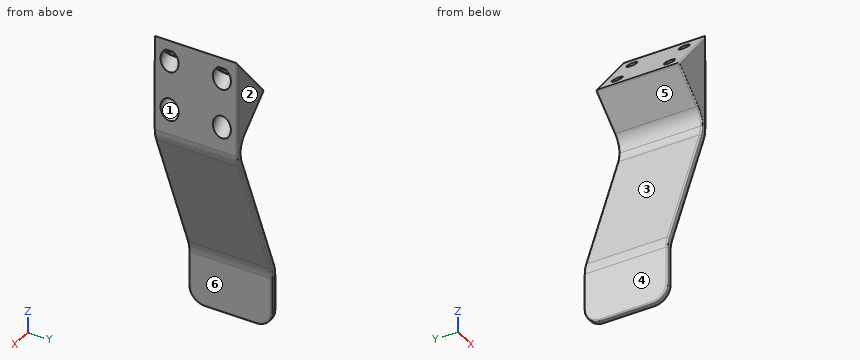
from build123d import *

# Parameters (mm, degrees)
SKETCH1_W           = 2
SKETCH1_H           = 25.4
SKETCH4_W           = 5
SKETCH4_H           = 25.4
CUT_EXTRUDE2_DEPTH  = 21
BOSS_EXTRUDE2_DEPTH = 25.4
BOSS_EXTRUDE4_DEPTH = 25.4
FILLET1_R           = 5
CUT_EXTRUDE3_DEPTH  = 26.4
SKETCH9_R           = 1.6
CUT_EXTRUDE4_DEPTH  = 2
SKETCH10_R          = 2.75
CUT_EXTRUDE5_DEPTH  = 59.842249491
FILLET2_R           = 10
FILLET5_R           = 6
FILLET3_R           = 0.4


with BuildPart() as part:
    # Sweep1: sweep along a path in Sketch2
    with BuildLine(Plane(origin=(0, 0, 0), x_dir=(1, 0, 0), z_dir=(0, 1, 0))) as sweep1_path:
        Line((22, 0), (22, 57.2))
        Line((22, 57.2), (4, 103.2))
        Line((4, 103.2), (4, 121.2))
    # Sketch1 → Sweep1 (sweep)
    with BuildSketch(Plane.XY):
        with Locations((22, 0)):
            Rectangle(SKETCH1_W, SKETCH1_H)
    sweep(path=sweep1_path.line, transition=Transition.RIGHT)

    # Sketch4 → Cut-Extrude2 (cut, through all)
    with BuildSketch(Plane(origin=(23, 0, 0), x_dir=(0, 0, -1), z_dir=(1, 0, 0))):
        with Locations((2.5, 0)):
            Rectangle(SKETCH4_W, SKETCH4_H)
    extrude(amount=-CUT_EXTRUDE2_DEPTH, mode=Mode.SUBTRACT)

    # Sketch5 → Boss-Extrude2 (add, through all)
    with BuildSketch(Plane.XZ.offset(12.7)):
        Polygon((21, -42.561313548), (21, -28.015116906), (9, -42.561313548), align=None)
    extrude(amount=-BOSS_EXTRUDE2_DEPTH)

    # Sketch6 → Boss-Extrude4 (add, through all)
    with BuildSketch(Plane.XZ.offset(12.7)):
        Polygon((9, -42.561313548), (21, -52.460808484), (21, -42.561313548), align=None)
    extrude(amount=-BOSS_EXTRUDE4_DEPTH)

    # Fillet1
    fillet1_edges = [part.edges().sort_by_distance(p)[0] for p in [
        (4, -12.7, -121.2),
        (4, 12.7, -121.2),
    ]]
    fillet(fillet1_edges, radius=FILLET1_R)

    # Sketch8 → Cut-Extrude3 (cut, through all)
    with BuildSketch(Plane.XZ.offset(12.7)):
        Polygon((23, -25.590750799), (23, -5), (21, -5), (21, -28.015116906), align=None)
    extrude(amount=-CUT_EXTRUDE3_DEPTH, mode=Mode.SUBTRACT)

    # Sketch9 → Cut-Extrude4 (cut)
    with BuildSketch(Plane(origin=(26.248041717, 0, -21.653529673), x_dir=(0.636363636, 0, 0.771389216), z_dir=(-0.771389216, 0, 0.636363636))):
        with Locations((-22.104065555, 8)):
            Circle(SKETCH9_R)
        with Locations((-22.104065555, -8)):
            Circle(SKETCH9_R)
        with Locations((-10.104065555, -8)):
            Circle(SKETCH9_R)
        with Locations((-10.104065555, 8)):
            Circle(SKETCH9_R)
    extrude(amount=-CUT_EXTRUDE4_DEPTH, mode=Mode.SUBTRACT)

    # Sketch10 → Cut-Extrude5 (cut, through all)
    with BuildSketch(Plane(origin=(27.790820149, 0, -22.926256946), x_dir=(0.636363636, 0, 0.771389216), z_dir=(-0.771389216, 0, 0.636363636))):
        with Locations((-22.104065555, 8)):
            Circle(SKETCH10_R)
        with Locations((-10.104065555, 8)):
            Circle(SKETCH10_R)
        with Locations((-10.104065555, -8)):
            Circle(SKETCH10_R)
        with Locations((-22.104065555, -8)):
            Circle(SKETCH10_R)
    extrude(amount=-CUT_EXTRUDE5_DEPTH, mode=Mode.SUBTRACT)

    # Fillet2
    fillet2_edges = [part.edges().sort_by_distance(p)[0] for p in [
        (23, 0, -57.388686452),
        (21, 0, -57.011313548),
        (3, 0, -103.011313548),
        (5, 0, -103.388686452),
    ]]
    fillet(fillet2_edges, radius=FILLET2_R)

    # Fillet5
    fillet5_edges = [part.edges().sort_by_distance(p)[0] for p in [
        (21, 0, -52.460808484),
    ]]
    fillet(fillet5_edges, radius=FILLET5_R)

    # Fillet3
    fillet3_edges = [part.edges().sort_by_distance(p)[0] for p in [
        (5, -12.7, -110.737775488),
        (5, 12.7, -110.737775488),
        (14, 12.7, -80.388686452),
        (14, -12.7, -80.388686452),
        (3, -12.7, -110.549089035),
        (3, 12.7, -110.549089035),
        (23, 12.7, -40.546286364),
        (12, 12.7, -80.011313548),
        (22.826603634, 12.7, -57.355968907),
        (3.173396366, 12.7, -103.044031093),
        (12, -12.7, -80.011313548),
        (23, -12.7, -40.546286364),
        (22.826603634, -12.7, -57.355968907),
        (3.173396366, -12.7, -103.044031093),
        (5.173396366, -12.7, -103.421403997),
        (5.173396366, 12.7, -103.421403997),
        (20.787013978, 12.7, -57.177339033),
        (20.787013978, -12.7, -57.177339033),
        (20.474647805, -12.7, -52.838617841),
        (20.474647805, 12.7, -52.838617841),
        (16, 12.7, -34.076032173),
        (9, 0, -42.561313548),
        (16, -12.7, -34.076032173),
        (13.907448432, 12.7, -46.609751957),
        (13.907448432, -12.7, -46.609751957),
        (5, 0, -121.2),
        (5, 11.235533906, -119.735533906),
        (5, -11.235533906, -119.735533906),
        (3, 0, -121.2),
        (3, 11.235533906, -119.735533906),
        (3, -11.235533906, -119.735533906),
    ]]
    fillet(fillet3_edges, radius=FILLET3_R)


solid = part.part
The listing builds one solid part. Answer for the finished solid, in the listing's coordinates (mm). Face numbers are marked on the shaded views. A direction names the side the tool comes from. Give positions to 0.01 mm unless a question says otherwise; leave off trailing zeros. Put each result on its own line as item: value.
Item 1: For a pull along Y with two mould halves and no side action, classify the marked faces 1, 2 and 3 as released by +Y, released by -Y, zero draft, split by the parting line, or undercut.
Established:
face 1: undercut
face 2: released by +Y
face 3: zero draft
Item 2: Given P1, Ø2, axis at y = -6, z = -62, coming from the -X side; P2, Ø5, axis at y = -9.5, z = -105, coming from the +X side; P3, Ø8, axis at y = 2, z = -116.5, coming from the +X side, each flat-ended and moving along its own axis, determine where each tip first touches the part or whether it passes through.
Established:
P1: stops at x = 18.66
P2: stops at x = 5.39
P3: stops at x = 5
Item 3: For the marked faces 4, 5 and 6, determine the directions among +Z, -Z, +X, -X, +Y, -Y from which every point of the face is accessible in a straight line to the end or side of a thin tool.
Established:
face 4: +Z, -Z, -X, +Y, -Y
face 5: -X, +Y, -Y
face 6: -Z, +X, +Y, -Y
Item 4: Straight lines are drawn through the part: line 1 (Y direction, x = 17, z = -42.5); line 2 (X direction, y = -8.75, z = -117); line 3 (X direction, y = 4.5, z = -42.5). For each, find the intervals that lie inside material, in ascending order.
Established:
line 1: y = -12.7 to -10.75, -5.25 to 5.25, 10.75 to 12.7
line 2: x = 3 to 5
line 3: x = 9.16 to 23
